Model file for the job. Use its own axes, mm. Face numbers are marked on the shaded views. A direction names the side the tool comes from. Coordinates: 2 decimals unless noted, no trailing zeros. Order: outer loops, then holes, each group sorted by start corner. A loop starts at its lowest first (then second) coordinate and runs counter-clockwise, first axis right, second up. Notation, with made-up numbers: (-5.5, -12) -> (42.5, -12) arc R26 ccw to (42.5, 19) -> close; hole circle Ø1 at (-19, 30). An arc over 180 degrees is marked (long way). Write item = value, one per line. Start each with the question number.
Q1. Cut at A-A, the plane z = 3.9. List the corners of the cut face in (x, y).
Q2. Flat gauge pin, fed straight in: pin 1 (3 mm diameter, centred on x = -3, y = 4, fed in from +Z). Where does the tip first touch, or does it go through?
Q3. Wall check: line 1 (Y direction, x = -5, z = 2.25); line 2 (X direction, y = 2, z = 2.15); line 3 (Z direction, x = -2.75, y = 5.25). Give the ranges that are in metal, low to high. Write a range as from..to.
Q4. Cut at C-C, the plane y = 3.5. List the corners of the cut face in (x, z).
Q5. 3-axis set-ups, long thin cutter, end or side, ignore diameter. For the marked faces 5 and 6: which of +Z, -Z, +X, -X, +Y, -Y reach the whole face in a straight line?
Q6. Cut at B-B, the plane x = -4.75. List the corners of the cut face in (y, z).
Q7. Cut at D-D, the plane y = 5.5. List the corners of the cut face in (x, z), plus the area to 3 significant figures.
Q8. Mould opens along Y. For the marked faces 1, 2, 3 and 4 say: +Y half, -Y half, draft (parallel to the pull), parting line (faces both ways), or undercut.
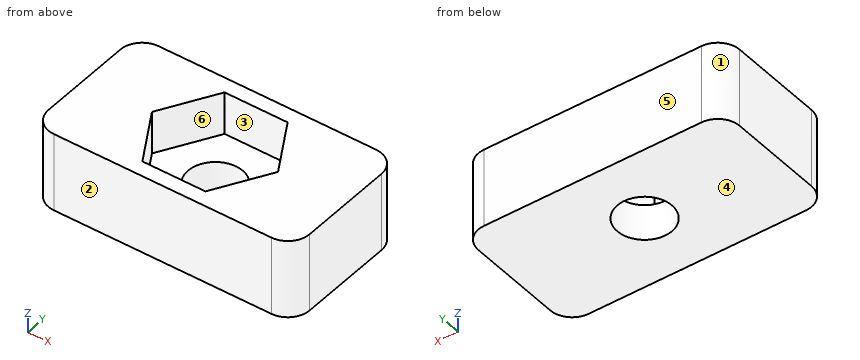
from build123d import *

# Parameters (mm, degrees)
F0_W     = 15.1892
F0_H     = 8.0899
F1_DEPTH = 4.572
F3_DEPTH = 2.4892
F4_R     = 1.5875
F5_DEPTH = 25.4
F6_R     = 1.27


with BuildPart() as f1:
    # F0 (on Top) → F1 (new body)
    with BuildSketch(Plane.XY):
        with Locations((-3.466585, 2.935039)):
            Rectangle(F0_W, F0_H)
    extrude(amount=F1_DEPTH)

    # F2 (on face) → F3 (cut)
    with BuildSketch(Plane.XY.offset(4.572)):
        Polygon((-1.633498, -0.239961), (0.199589, 2.935039), (-1.633498, 6.110039), (-5.299672, 6.110039), (-7.132759, 2.935039), (-5.299672, -0.239961), align=None)
    extrude(amount=-F3_DEPTH, mode=Mode.SUBTRACT)

    # F4 (on face) → F5 (cut)
    with BuildSketch(Plane.XY.offset(2.0828)):
        with Locations((-3.443841, 2.935039)):
            Circle(F4_R)
    extrude(amount=-F5_DEPTH, mode=Mode.SUBTRACT)

    # F6
    f6_edges = [f1.edges().sort_by_distance(p)[0] for p in [
        (4.128015, -1.109911, 2.286),
        (-11.061185, -1.109911, 2.286),
        (-11.061185, 6.979989, 2.286),
        (4.128015, 6.979989, 2.286),
    ]]
    fillet(f6_edges, radius=F6_R)


solid = f1.part
Here are the results:
q1.outline = (-11.06, 0.16) arc R1.27 ccw to (-9.79, -1.11) -> (2.86, -1.11) arc R1.27 ccw to (4.13, 0.16) -> (4.13, 5.71) arc R1.27 ccw to (2.86, 6.98) -> (-9.79, 6.98) arc R1.27 ccw to (-11.06, 5.71) -> close; hole (-7.13, 2.94) -> (-5.3, -0.24) -> (-1.63, -0.24) -> (0.2, 2.94) -> (-1.63, 6.11) -> (-5.3, 6.11) -> close
q2.pin_1 = 2.08
q3.line_1 = -1.11..-0.24, 6.11..6.98
q3.line_2 = -11.06..-6.59, -0.34..4.13
q3.line_3 = 0..2.08
q4.outline = (-11.06, 0) -> (-4.93, 0) -> (-4.93, 2.08) -> (-6.81, 2.08) -> (-6.81, 4.57) -> (-11.06, 4.57) -> close; (-1.96, 0) -> (4.13, 0) -> (4.13, 4.57) -> (-0.13, 4.57) -> (-0.13, 2.08) -> (-1.96, 2.08) -> close
q5.face_5 = +Z, -Z, +X, -X, +Y
q5.face_6 = +Z
q6.outline = (-1.11, 0) -> (2.03, 0) -> (2.03, 2.08) -> (-0.24, 2.08) -> (-0.24, 4.57) -> (-1.11, 4.57) -> close; (3.84, 0) -> (6.98, 0) -> (6.98, 4.57) -> (6.11, 4.57) -> (6.11, 2.08) -> (3.84, 2.08) -> close
q7.outline = (-11.06, 0) -> (4.13, 0) -> (4.13, 4.57) -> (-1.28, 4.57) -> (-1.28, 2.08) -> (-5.65, 2.08) -> (-5.65, 4.57) -> (-11.06, 4.57) -> close
q7.area = 58.6 mm²
q8.face_1 = +Y half
q8.face_2 = -Y half
q8.face_3 = undercut
q8.face_4 = draft
